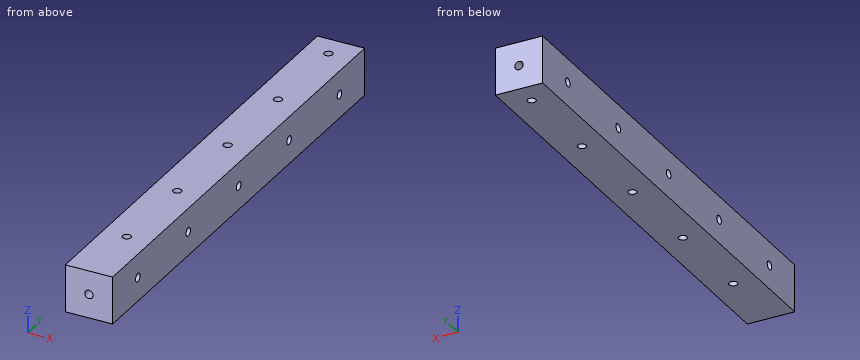
from build123d import *

# Parameters (mm, degrees)
SKETCH1_W                           = 12.7
SKETCH1_H                           = 12.7
BOSS_EXTRUDE1_DEPTH                 = 127
F_4_40_TAPPED_HOLE1_D               = 2.2606
F_4_40_TAPPED_HOLE1_DEPTH           = 7.6
F_4_40_TAPPED_HOLE1_TIP             = 0.679152758
F_4_40_TAPPED_HOLE1_ON_FACE_2_D     = 2.2606
F_4_40_TAPPED_HOLE1_ON_FACE_2_DEPTH = 7.6
F_4_40_TAPPED_HOLE1_ON_FACE_2_TIP   = 0.679152758
F_4_40_TAPPED_HOLE2_D               = 2.2606
LPATTERN1_COUNT                     = 5
LPATTERN1_PITCH                     = 25.4
F_4_40_TAPPED_HOLE3_OUTLINE_R       = 1.1303
F_4_40_TAPPED_HOLE3_DEPTH           = 12.7
LPATTERN2_COUNT                     = 5
LPATTERN2_PITCH                     = 25.4


# Read off the part's stored shape, not the designer's step: #4-40 Tapped Hole3
with BuildPart() as part:
    # Sketch1 → Boss-Extrude1 (new body)
    with BuildSketch(Plane(origin=(0, 0, 0), x_dir=(1, 0, 0), z_dir=(0, 1, 0))):
        with Locations((6.35, -6.35)):
            Rectangle(SKETCH1_W, SKETCH1_H)
    extrude(amount=BOSS_EXTRUDE1_DEPTH)

    # #4-40 Tapped Hole1
    with Locations(Plane(origin=(6.35, 127, 6.35), x_dir=(0, 0, 1), z_dir=(0, 1, 0))):
        with Locations((0, 0)):
            Hole(F_4_40_TAPPED_HOLE1_D / 2, depth=F_4_40_TAPPED_HOLE1_DEPTH)
            with Locations((0, 0, -(F_4_40_TAPPED_HOLE1_DEPTH + F_4_40_TAPPED_HOLE1_TIP / 2))):  # 118° drill point
                Cone(0, F_4_40_TAPPED_HOLE1_D / 2, F_4_40_TAPPED_HOLE1_TIP, mode=Mode.SUBTRACT)

    # #4-40 Tapped Hole1 on face 2
    with Locations(Plane(origin=(6.35, 0, 6.35), x_dir=(0, 0, -1), z_dir=(0, -1, 0))):
        with Locations((0, 0)):
            Hole(F_4_40_TAPPED_HOLE1_ON_FACE_2_D / 2, depth=F_4_40_TAPPED_HOLE1_ON_FACE_2_DEPTH)
            with Locations((0, 0, -(F_4_40_TAPPED_HOLE1_ON_FACE_2_DEPTH + F_4_40_TAPPED_HOLE1_ON_FACE_2_TIP / 2))):  # 118° drill point
                Cone(0, F_4_40_TAPPED_HOLE1_ON_FACE_2_D / 2, F_4_40_TAPPED_HOLE1_ON_FACE_2_TIP, mode=Mode.SUBTRACT)

    # #4-40 Tapped Hole2 (through all)
    with Locations(Plane(origin=(6.35, 120.65, 0), x_dir=(-1, 0, 0), z_dir=(0, 0, -1))):
        with Locations((0, 0)):
            f_4_40_tapped_hole2 = Hole(F_4_40_TAPPED_HOLE2_D / 2)

    # LPattern1: #4-40 Tapped Hole2 ×5
    with Locations(*[(0, -i * LPATTERN1_PITCH, 0) for i in range(1, LPATTERN1_COUNT)]):
        add(f_4_40_tapped_hole2, mode=Mode.SUBTRACT)

    # #4-40 Tapped Hole3 outline → #4-40 Tapped Hole3 (cut)
    with BuildSketch(Plane.YZ):
        with Locations((114.3, 6.35)):
            Circle(F_4_40_TAPPED_HOLE3_OUTLINE_R)
    f_4_40_tapped_hole3 = extrude(amount=F_4_40_TAPPED_HOLE3_DEPTH, mode=Mode.SUBTRACT)

    # LPattern2: #4-40 Tapped Hole3 ×5
    with Locations(*[(0, -i * LPATTERN2_PITCH, 0) for i in range(1, LPATTERN2_COUNT)]):
        add(f_4_40_tapped_hole3, mode=Mode.SUBTRACT)


solid = part.part
The listing builds one solid part. Answer for the finished solid, in the listing's coordinates (mm). Give positions to 0.01 mm unless a question says otherwise; leave off trailing zeros. Loops run counter-clockwise (first coordinate to the right, second up) from the corner with the lowest first, then second, coordinate; pieces in that order, holes last.
Item 1: A cutting plane is placed at A-A (y = 63.5). Give the vertices of the cut face in (x, z).
Derived:
outline: (0, 0) - (12.7, 0) - (12.7, 5.22) - (0, 5.22) - close; (0, 7.48) - (12.7, 7.48) - (12.7, 12.7) - (0, 12.7) - close
Item 2: Each of these flat-tipped pins is pushed along its axis until it touches: pin 1 Ø1.8 at (x, y) = (6.35, 120.65) entering from -Z; pin 2 Ø2 at (x, z) = (6.35, 6.35) entering from +Y. Where does it stop, or does it pass through?
Derived:
pin 1: passes through
pin 2: stops at y = 119.32
Item 3: Find the intervals of material crossed by line 1 along Y through (x, z) = (6.35, 4.75); line 2 along Z through (x, y) = (6.35, 125.25), in increasing order.
Derived:
line 1: y = 0 to 17.92, 20.18 to 43.32, 45.58 to 68.72, 70.98 to 94.12, 96.38 to 119.52, 121.78 to 127
line 2: z = 0 to 5.22, 7.48 to 12.7
